Read the model definition and answer for the solid it produces. Units are mm, in the model's axes. A direction names the side the tool comes from. Coordinates: 2 decimals unless noted, no trailing zeros. Order: outer loops, then holes, each group sorted by start corner. A loop starts at its lowest first (then second) coordinate and runs counter-clockwise, first axis right, second up.
```python
from build123d import *

# Parameters (mm, degrees)
BOSS_EXTRUDE1_DEPTH = 7.32


with BuildPart() as part:
    # Sketch1 → Boss-Extrude1 (new body)
    with BuildSketch(Plane.XY):
        Polygon((0, 10.779129526), (-9.335, 5.389564763), (-9.335, -5.389564763), (0, -10.779129526), (9.335, -5.389564763), (9.335, 5.389564763), align=None)
    extrude(amount=BOSS_EXTRUDE1_DEPTH)

    # Sketch2 → Revolve1 (revolve)
    with BuildSketch(Plane(origin=(0, 0, 0), x_dir=(0, 0, -1), z_dir=(1, 0, 0))):
        with BuildLine():
            Line((0, 0), (0, 6.6))
            ThreePointArc((0, 6.6), (0.175735931, 6.175735931), (0.6, 6))
            Line((0.6, 6), (199.1, 6))
            Line((199.1, 6), (200, 5.1))
            Line((200, 5.1), (200, 0))
            Line((200, 0), (0, 0))
        make_face()
    revolve(axis=Axis((0, 0, 0), (0, 0, -1)))

    # Sketch3 → Cut-Revolve1 (revolve, cut)
    with BuildSketch(Plane(origin=(0, 0, 0), x_dir=(0, 0, -1), z_dir=(1, 0, 0))):
        Polygon((-7.32, 10.779129526), (-6.48623143, 10.779129526), (-7.32, 9.335), align=None)
        Polygon((-0.15, 10.779129526), (-0.15, 8.78660254), (0, 8.7), (0, 10.779129526), align=None)
    revolve(axis=Axis((0, 0, 12.204941078), (0, 0, -1)), mode=Mode.SUBTRACT)


solid = part.part
```
1) Which of the six approach directions +Z, -Z, +X, -X, +Y, -Y give full straight-line access (tool end or side, diameter ignored) to faces 1 (the flat face through (0, 0, 7.32)), 2 (the flat face through (1, 9, 0.15))?
A:
face 1: +Z, +X, -X, +Y, -Y
face 2: -Z
2) Flat-ended cylindrical pins translate along their axes: pin 1 Ø3 at (x, z) = (3, -27) entering from -Y; pin 2 Ø1 at (x, z) = (3, -53) entering from +Y; pin 3 Ø4 at (x, z) = (-3.5, -89) entering from +Y; pin 4 Ø2 at (x, z) = (-7.5, -137) entering from -Y. Find the tip coordinate at first contact, or state that the pin passes through.
A:
pin 1: stops at y = -5.81
pin 2: stops at y = 5.45
pin 3: stops at y = 5.81
pin 4: passes through
3) Straight lines are drawn through the part: line 1 (X direction, y = -0.25, z = -167.5); line 2 (Z direction, x = -8, y = -4); line 3 (Z direction, x = 4.75, y = -6.25). For each, find the intervals that lie inside material, in ascending order.
A:
line 1: x = -5.99 to 5.99
line 2: z = 0.15 to 7.32
line 3: z = 0 to 7.32
4) A cutting plane is placed at A-A, the plane z = -141. Determine the outline of the cut face in (x, y).
A:
outline: circle Ø12 at (0, 0)
